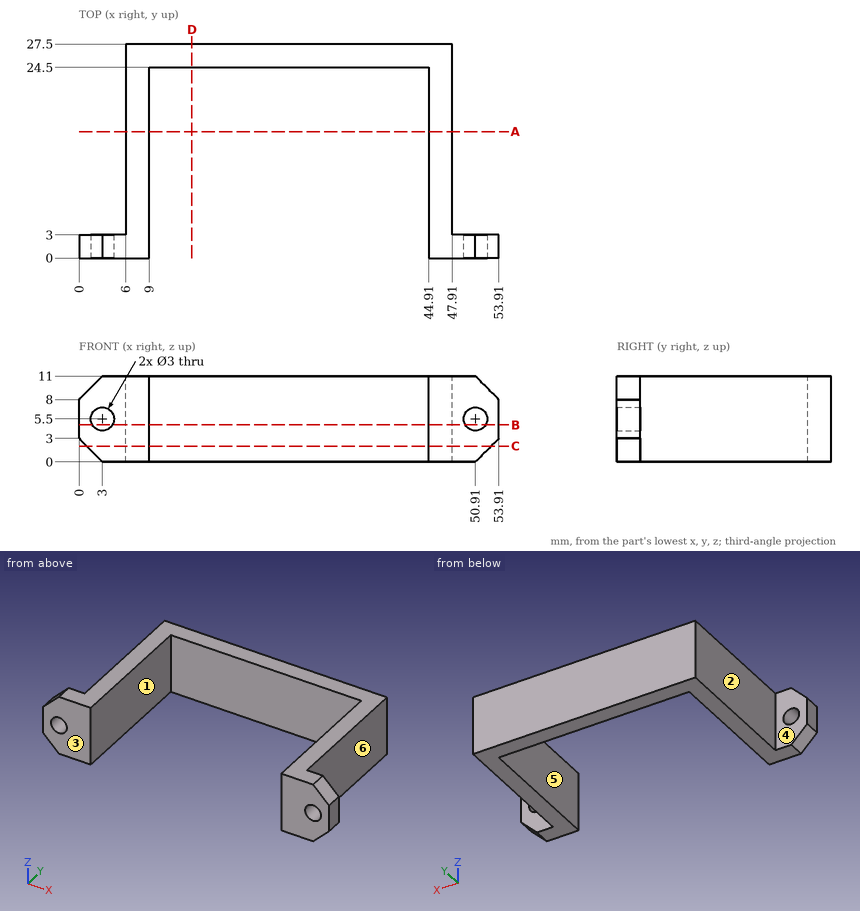
Could you check a few things on this drawing? It's one solid part, dimensions in mm from its lowest x, y, z. A direction names the side the tool comes from. Round coordinates to 2 decimals unless told otherwise and drop trailing zeros. Write each loop counter-clockwise with the first axis right and the second up, starting at its lowest first coordinate (ties: lowest second). Pieces come first, ordered by that corner, then holes. Notation, with made-up numbers: (-39.5, 28) -> (-31.5, 28) arc R25 ccw to (-31.5, 43) -> close; hole circle Ø4 at (-16.5, 54). An arc over 180 degrees is marked (long way). Use one line per item in the form item = value. Start each with the question number.
Q1. If I drill on probe 1 along X at (y, z) = (12.25, 5.25); probe 2 along X at (y, z) = (1.75, 7.5); probe 3 along Y at (x, z) = (3.5, 3.25), over which ranges is the centre line in solid material (lowest first)? Write a range as [from, to].
Q2. We'd pull the mould along X, two halves only. Please class the marked faces 4, 5 and 6: +X half, -X half, draft (parallel to the pull), parting line (faces both ways), or undercut.
Q3. Imagine slicing it at B-B (z = 4.75). Please give me the cut outline in (x, y).
Q4. I'm going to push flat-ended pins straight in: P1, Ø2.5, axis at x = 50.91, z = 5.5, coming from the -Y side; P2, Ø5, axis at y = 21, z = 6.5, coming from the -X side; P3, Ø5.5, axis at y = 16, z = 7, coming from the +X side; P4, Ø2, axis at x = 36.5, z = 3, coming from the -Y side. Where does each tip first touch, or does it pass through?
Q5. Imagine slicing it at D-D (x = 14.5). Please give me the cut outline in (y, z).
Q6. Imagine slicing it at C-C (z = 2). Please give me the cut outline in (x, y), then the cut area to 3 significant figures.
Q7. Which directions (+Z, -Z, +X, -X, +Y, -Y) give clear straight access to the entire face, cutting with the end or side of a thin tool? Please do the marked faces 1, 2 and 3.
Q8. Imagine slicing it at A-A (y = 16.25). Please give me the cut outline in (x, z).
Worked out:
q1.probe_1 = [6, 9], [44.91, 47.91]
q1.probe_2 = [0, 9], [44.91, 53.91]
q1.probe_3 = [0, 3]
q2.face_4 = draft
q2.face_5 = undercut
q2.face_6 = +X half
q3.outline = (0, 0) -> (1.7, 0) -> (1.7, 3) -> (0, 3) -> close; (4.3, 0) -> (9, 0) -> (9, 24.5) -> (44.91, 24.5) -> (44.91, 0) -> (49.61, 0) -> (49.61, 3) -> (47.91, 3) -> (47.91, 27.5) -> (6, 27.5) -> (6, 3) -> (4.3, 3) -> close; (52.21, 0) -> (53.91, 0) -> (53.91, 3) -> (52.21, 3) -> close
q4.P1 = through
q4.P2 = 6
q4.P3 = 47.91
q4.P4 = 24.5
q5.outline = (24.5, 0) -> (27.5, 0) -> (27.5, 11) -> (24.5, 11) -> close
q6.outline = (1, 0) -> (9, 0) -> (9, 24.5) -> (44.91, 24.5) -> (44.91, 0) -> (52.91, 0) -> (52.91, 3) -> (47.91, 3) -> (47.91, 27.5) -> (6, 27.5) -> (6, 3) -> (1, 3) -> close
q6.area = 303 mm^2
q7.face_1 = +Z, -Z, -Y
q7.face_2 = +Z, -Z, -X, +Y
q7.face_3 = +Z, -Z, +X, -X, -Y
q8.outline = (6, 0) -> (9, 0) -> (9, 11) -> (6, 11) -> close; (44.91, 0) -> (47.91, 0) -> (47.91, 11) -> (44.91, 11) -> close
